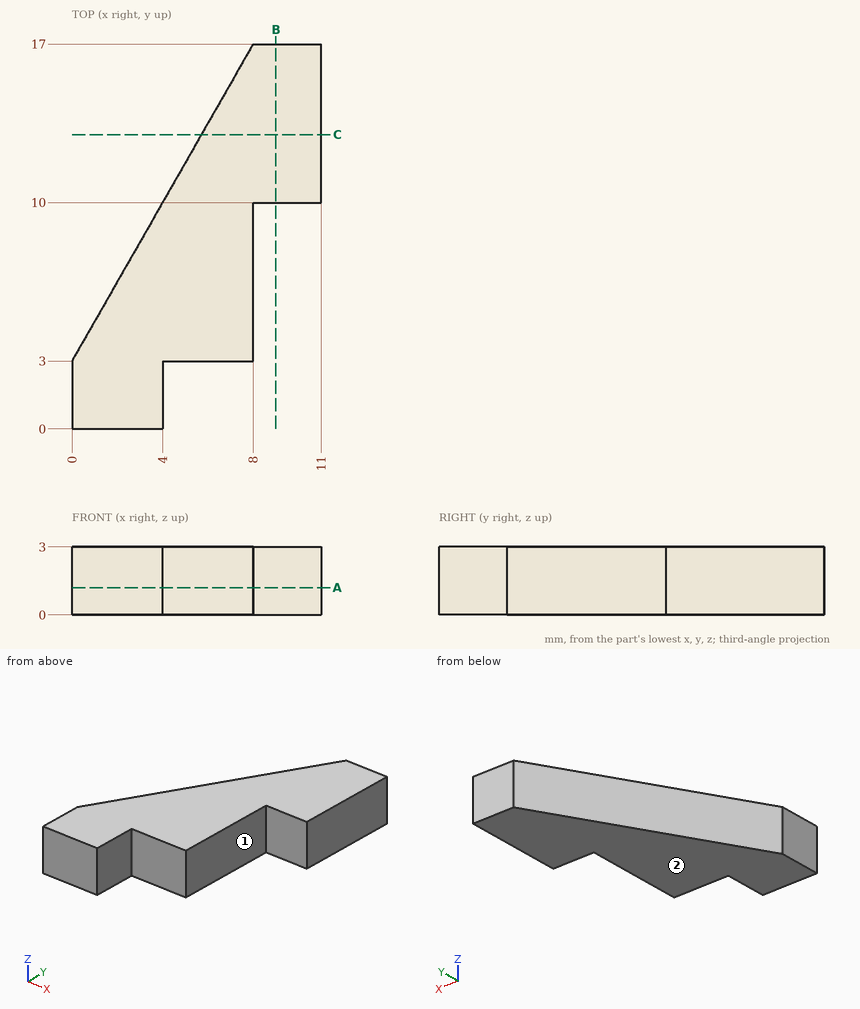
The figure shows three views and two pictorial views of one solid part (mm, origin at its lowest corner). Answer the questions. A direction names the side the tool comes from. Give positions to 0.01 mm unless a question says otherwise; leave off trailing zeros. Order: outer loops, then holes, each group sorted by start corner. A loop starts at its lowest first (then second) coordinate and runs counter-clockwise, first axis right, second up. Notation, with made-up numbers: M -11,81.25 L 34,81.25 A15 cw 34,87.25 Z; hole C -10.75,73 d2. An arc over 180 degrees is marked long. Return JSON: item names as keys, results as strings.
1) Section B-B, the plane x = 9 is taken. Write down the section's boundary in (y, z), plus the area to 3 significant figures.
Resolved:
{"outline": "M 10,0 L 17,0 L 17,3 L 10,3 Z", "area": "21.0 mm^2"}
2) Each of these flat-tipped pins is pushed along its axis until it touches: pin 1 (1.5 mm diameter, centred on y = 7.5, z = 2, fed in from +X); pin 2 (1.5 mm diameter, centred on x = 6, z = 2, fed in from -Y); pin 3 (3 mm diameter, centred on x = 2.5, y = 13.5, fed in from +Z); pin 4 (0.9 mm diameter, centred on x = 9.5, z = 1, fed in from -Y). Where does it stop, or does it pass through?
Resolved:
{"pin 1": "x = 8", "pin 2": "y = 3", "pin 3": "through", "pin 4": "y = 10"}
3) Section C-C, the plane y = 13 is taken. Write down the section's boundary in (x, z), plus the area to 3 significant figures.
Resolved:
{"outline": "M 5.71,0 L 11,0 L 11,3 L 5.71,3 Z", "area": "15.9 mm^2"}
4) Section A-A, the plane z = 1.2 is taken. Write down the section's boundary in (x, y), plus the area to 3 significant figures.
Resolved:
{"outline": "M 0,0 L 4,0 L 4,3 L 8,3 L 8,10 L 11,10 L 11,17 L 8,17 L 0,3 Z", "area": "89.0 mm^2"}
5) Straight lines are drawn through the part: line 1 along Y through (x, z) = (8.5, 2.65); line 2 along X through (y, z) = (5.25, 1.85); line 3 along X through (y, z) = (11.5, 2.35). For each, find the intervals that lie inside material, in ascending order. Write a range as [from, to].
Resolved:
{"line 1": "[10, 17]", "line 2": "[1.29, 8]", "line 3": "[4.86, 11]"}
6) A tool of negligible diameter and unlimited length cuts with its end or side. For the marked faces 1 and 2, from which of +Z, -Z, +X, -X, +Y, -Y can it reach the whole face along a straight path? Write none if from no direction.
Resolved:
{"face 1": "+Z, -Z, +X, -Y", "face 2": "-Z, +X, -X, +Y, -Y"}
